```python
from build123d import *

# Parameters (mm, degrees)
SKETCH_W   = 140
SKETCH_H   = 60
SKETCH_R   = 2.5
SKETCH_R_2 = 1
PAD_DEPTH  = 1.8


with BuildPart() as part:
    # Sketch → Pad (new body)
    with BuildSketch(Plane.XY):
        with Locations((68.5, 39.5)):
            Rectangle(SKETCH_W, SKETCH_H)
        with Locations((28.5, 14.5)):
            Circle(SKETCH_R, mode=Mode.SUBTRACT)
        with Locations((108.5, 14.5)):
            Circle(SKETCH_R, mode=Mode.SUBTRACT)
        with Locations((8.5, 24.5)):
            Circle(SKETCH_R, mode=Mode.SUBTRACT)
        with Locations((48.5, 24.5)):
            Circle(SKETCH_R, mode=Mode.SUBTRACT)
        with Locations((88.5, 24.5)):
            Circle(SKETCH_R, mode=Mode.SUBTRACT)
        with Locations((8.5, 44.5)):
            Circle(SKETCH_R, mode=Mode.SUBTRACT)
        with Locations((48.5, 44.5)):
            Circle(SKETCH_R, mode=Mode.SUBTRACT)
        with Locations((88.5, 44.5)):
            Circle(SKETCH_R, mode=Mode.SUBTRACT)
        with Locations((28.5, 54.5)):
            Circle(SKETCH_R, mode=Mode.SUBTRACT)
        with Locations((68.5, 54.5)):
            Circle(SKETCH_R, mode=Mode.SUBTRACT)
        with Locations((108.5, 54.5)):
            Circle(SKETCH_R, mode=Mode.SUBTRACT)
        with Locations((88.5, 64.5)):
            Circle(SKETCH_R, mode=Mode.SUBTRACT)
        with Locations((48.5, 64.5)):
            Circle(SKETCH_R, mode=Mode.SUBTRACT)
        with Locations((8.5, 64.5)):
            Circle(SKETCH_R, mode=Mode.SUBTRACT)
        with Locations((28.5, 34.5)):
            Circle(SKETCH_R, mode=Mode.SUBTRACT)
        with Locations((68.5, 34.5)):
            Circle(SKETCH_R, mode=Mode.SUBTRACT)
        with Locations((108.5, 34.5)):
            Circle(SKETCH_R, mode=Mode.SUBTRACT)
        with Locations((68.5, 14.5)):
            Circle(SKETCH_R, mode=Mode.SUBTRACT)
        with Locations((128.5, 24.5)):
            Circle(SKETCH_R, mode=Mode.SUBTRACT)
        with Locations((128.5, 44.5)):
            Circle(SKETCH_R, mode=Mode.SUBTRACT)
        with Locations((128.5, 64.5)):
            Circle(SKETCH_R, mode=Mode.SUBTRACT)
        with Locations((68.5, 39.5)):
            Circle(SKETCH_R_2, mode=Mode.SUBTRACT)
    extrude(amount=PAD_DEPTH)


solid = part.part
```
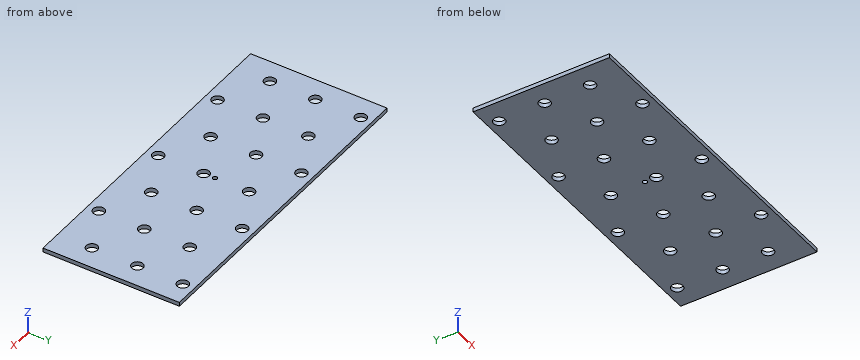
Could you check a few things on this model? Use its own coordinates, in mm. Coordinates: 2 decimals unless noted, no trailing zeros. Write each loop counter-clockwise with the first axis right and the second up, starting at its lowest first coordinate (ties: lowest second). Pieces come first, ordered by that corner, then holes. Notation, with made-up numbers: (22.5, 71) -> (32.5, 71) arc R18 cw to (32.5, 87) -> close; hole circle Ø7 at (51, 68.25). An arc over 180 degrees is marked (long way). One line per question, with ' | ' between items. Start each with the question number.
1. Please list where these lines run through material, in increasing order: line 1 along Y through (x, z) = (88.5, 0.6); line 2 along X through (y, z) = (66.5, 1.5); line 3 along Y through (x, z) = (69, 1.2).
2. If we section it at A-A (y = 24.5): Please give me the cut outline in (x, z).
3. If we section it at D-D (y = 14.5): Please give me the cut outline in (x, z).
4. If we section it at C-C (z = 1.15): Count the separate pieces of the cut face and the enclosed holes in it, and give its area (3 significant figures).
5. If we section it at B-B (x = 28.5): Please give me the cut outline in (y, z).
Return value:
1) line 1: y = 9.5 to 22, 27 to 42, 47 to 62, 67 to 69.5 | line 2: x = -1.5 to 7, 10 to 47, 50 to 87, 90 to 127, 130 to 138.5 | line 3: y = 9.5 to 12.05, 16.95 to 32.05, 36.95 to 38.63, 40.37 to 52.05, 56.95 to 69.5
2) outline: (-1.5, 0) -> (6, 0) -> (6, 1.8) -> (-1.5, 1.8) -> close; (11, 0) -> (46, 0) -> (46, 1.8) -> (11, 1.8) -> close; (51, 0) -> (86, 0) -> (86, 1.8) -> (51, 1.8) -> close; (91, 0) -> (126, 0) -> (126, 1.8) -> (91, 1.8) -> close; (131, 0) -> (138.5, 0) -> (138.5, 1.8) -> (131, 1.8) -> close
3) outline: (-1.5, 0) -> (26, 0) -> (26, 1.8) -> (-1.5, 1.8) -> close; (31, 0) -> (66, 0) -> (66, 1.8) -> (31, 1.8) -> close; (71, 0) -> (106, 0) -> (106, 1.8) -> (71, 1.8) -> close; (111, 0) -> (138.5, 0) -> (138.5, 1.8) -> (111, 1.8) -> close
4) separate pieces: 1 | enclosed holes: 22 | area: 7,980 mm²
5) outline: (9.5, 0) -> (12, 0) -> (12, 1.8) -> (9.5, 1.8) -> close; (17, 0) -> (32, 0) -> (32, 1.8) -> (17, 1.8) -> close; (37, 0) -> (52, 0) -> (52, 1.8) -> (37, 1.8) -> close; (57, 0) -> (69.5, 0) -> (69.5, 1.8) -> (57, 1.8) -> close
